Geometry: final body of the model. Coordinates: model frame, mm. A direction names the side the tool comes from. Give positions to 0.01 mm unless a question says otherwise; leave off trailing zeros. Write each loop counter-clockwise with the first axis right and the second up, starting at its lowest first coordinate (ties: lowest second). Pieces come first, ordered by that corner, then holes. Notation, with made-up numbers: M -10,-37.75 L 41,-37.75 A15 ccw 41,-14.75 Z; hole C 50,36.25 d9. An arc over 180 degrees is marked long. Use a Markdown table: item, result. Add a question column.
1) Draft query along Y for faces 1 (the flat face through (-11.533, -21, 5)), 2 (the cylindrical face through (-16.752, -5.182, 4.944)), 3 (the flat face through (-25, 0, 5)), 4 (the flat face through (8, -24.803, 5)). Return one class per face: +Y half, -Y half, draft (parallel to the pull), parting line (faces both ways), or undercut.
2) Pin query (flat end, axial travel): pin 1 (3 mm diameter, centred on x = -12.5, z = 6.5, fed in from -Y); pin 2 (2 mm diameter, centred on y = -21, z = 4.5, fed in from +X); pin 3 (1.3 mm diameter, centred on x = 45, z = 6.5, fed in from -Y); pin 4 (3.5 mm diameter, centred on y = -16.5, z = 6, fed in from -X). Return the tip coordinate at first contact, or that it passes through.
3) Set-up query: faces 5 (the flat face through (-16, -17.803, 5)), 6 (the flat face through (46.917, -3, 5)), 7 (the flat face through (-29.983, -3, 5)), 8 (the flat face through (-10.31, -9.026, 4.93)), 9 (the flat face through (37.792, -16, 5)). Return all of +Z, -Z, +X, -X, +Y, -Y with unobstructed straight access to the full face (end or side cutting, diameter ignored); none if empty.
4) Line query: line 1 (X direction, y = -6, z = 3); line 2 (Y direction, x = -26, z = 1.5); line 3 (X direction, y = -5.75, z = 7.5). Output: solid intervals per line, ascending.
5) Section A-A on y = -16.5. Return the cut outline in (x, z).
6) Section C-C on y = -19.75. Return the cut outline in (x, z), then the cut area to 3 significant figures.
7) Section B-B on x = 3. Return the cut outline in (y, z).
```python
from build123d import *

# Parameters (mm, degrees)
F1_DEPTH = 10
F2_R     = 1
F3_R     = 1


with BuildPart() as f1:
    # F0 (on Top) → F1 (new body)
    with BuildSketch(Plane.XY):
        with BuildLine():
            Line((-20.85751, -17.803463), (-11.53251, -17.803463))
            Line((-11.53251, -17.803463), (-1.53251, -17.803463))
            Line((-1.53251, -17.803463), (-19.335973, 0))
            Line((-19.335973, 0), (-25.98251, 0))
            Line((-25.98251, 0), (-29.98251, 0))
            Line((-29.98251, 0), (-29.98251, -6.5))
            Line((-29.98251, -6.5), (-25.674472, -6.5))
            ThreePointArc((-25.674472, -6.5), (-16.660227, -5.309177), (-20.85751, -13.375))
            Line((-20.85751, -13.375), (-20.85751, -16.5))
            Line((-20.85751, -16.5), (-20.85751, -17.803463))
        make_face()
        Polygon((-1.53251, -17.803463), (-11.53251, -17.803463), (-11.53251, -24.803463), (8.46749, -24.803463), (8.46749, -17.803463), align=None)
        Polygon((18.46749, -17.803463), (8.46749, -17.803463), (8.46749, -24.803463), (28.46749, -24.803463), (28.46749, -17.803463), align=None)
        with BuildLine():
            Line((36.270953, 0), (18.46749, -17.803463))
            Line((18.46749, -17.803463), (28.46749, -17.803463))
            Line((28.46749, -17.803463), (37.79249, -17.720502))
            Line((37.79249, -17.720502), (37.79249, -13.375))
            ThreePointArc((37.79249, -13.375), (33.595207, -5.309177), (42.609452, -6.5))
            Line((42.609452, -6.5), (46.91749, -6.5))
            Line((46.91749, -6.5), (46.91749, 0))
            Line((46.91749, 0), (42.91749, 0))
            Line((42.91749, 0), (36.270953, 0))
        make_face()
    extrude(amount=F1_DEPTH)

    # F2
    f2_edges = [f1.edges().sort_by_distance(p)[0] for p in [
        (-16.660227, -5.309177, 10),
    ]]
    fillet(f2_edges, radius=F2_R)

    # F3
    f3_edges = [f1.edges().sort_by_distance(p)[0] for p in [
        (33.595207, -5.309177, 10),
        (-16.660227, -5.309177, 0),
        (33.595207, -5.309177, 0),
    ]]
    fillet(f3_edges, radius=F3_R)


solid = f1.part
```
Found:
| question | item | result |
|---|---|---|
| 1 | face 1 | draft |
| 1 | face 2 | undercut |
| 1 | face 3 | +Y half |
| 1 | face 4 | -Y half |
| 2 | pin 1 | y = -24.8 |
| 2 | pin 2 | x = 28.47 |
| 2 | pin 3 | y = -6.5 |
| 2 | pin 4 | x = -20.86 |
| 3 | face 5 | +Z, -Z, -X, -Y |
| 3 | face 6 | +Z, -Z, +X, +Y, -Y |
| 3 | face 7 | +Z, -Z, -X, +Y, -Y |
| 3 | face 8 | +Z, -Z, +Y |
| 3 | face 9 | +Z, -Z, +X, -Y |
| 4 | line 1 | -29.98 to -25.46, -16.25 to -13.34, 30.27 to 33.19, 42.4 to 46.92 |
| 4 | line 2 | -6.5 to 0 |
| 4 | line 3 | -29.98 to -25.33, -16.38 to -13.59, 30.52 to 33.32, 42.27 to 46.92 |
| 5 | outline | M -20.86,0 L -2.84,0 L -2.84,10 L -20.86,10 Z; M 19.77,0 L 37.79,0 L 37.79,10 L 19.77,10 Z |
| 6 | outline | M -11.53,0 L 28.47,0 L 28.47,10 L -11.53,10 Z |
| 6 | area | 400 mm² |
| 7 | outline | M -24.8,0 L -17.8,0 L -17.8,10 L -24.8,10 Z |
